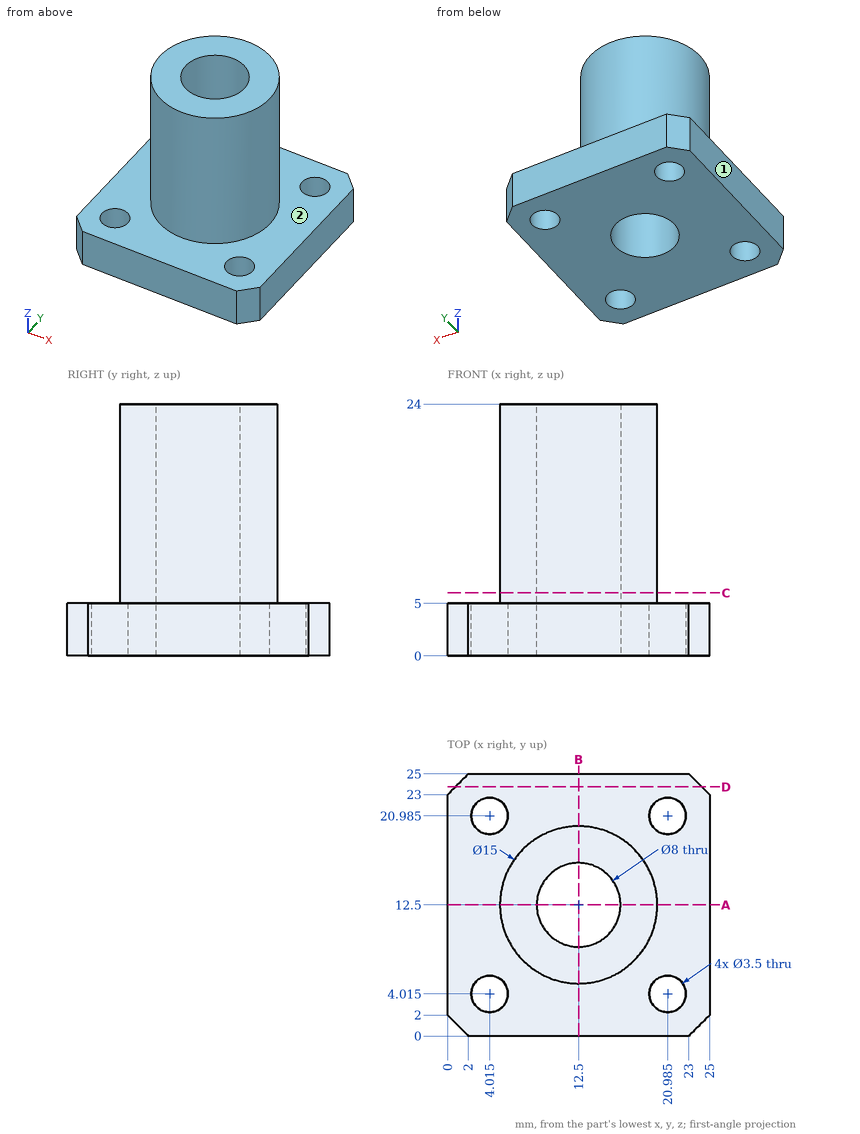
Could you check a few things on this drawing? It's one solid part, dimensions in mm from its lowest x, y, z. A direction names the side the tool comes from. Coordinates: 2 decimals unless noted, no trailing zeros. Order: outer loops, then holes, each group sorted by start corner. A loop starts at its lowest first (then second) coordinate and runs counter-clockwise, first axis right, second up. Notation, with made-up numbers: (-11.5, -10) - (-2.5, -10) arc R15 ccw to (-2.5, 16) - close; hole circle Ø9 at (-5, -8.5). An arc over 180 degrees is marked (long way). Answer as a JSON object with one key per item and string values. Group by question number.
Q1. Imagine slicing it at C-C (z = 6). Please give me the cut outline in (x, y), and give its area (3 significant figures).
Q2. On a 3-axis mill with a long thin cutter (end or side, diameter ignored), from which of +Z, -Z, +X, -X, +Y, -Y can I reach the whole of each face in a straight line? I mean the marked faces 1 and 2. Say none if no direction works.
Q3. I need wall thicknesses on line 1 (Y direction, x = 12.5, z = 13); line 2 (Z direction, x = 4.5, y = 15); line 3 (Y direction, x = 9.75, z = 6) (1 decimal). Which ranges of each line are inside material? Lowest first, please. Write a range as from..to.
Q4. Imagine slicing it at D-D (y = 23.75). Please give me the cut outline in (x, z).
Q5. Will these pins go through, and if not, where does the flat tip stop? P1, Ø5, axis at y = 6.5, z = 20.5, coming from the +X side; P2, Ø8, axis at x = 7.5, y = 5.5, coming from the -Z side; P3, Ø2, axis at x = 15.5, z = 12.5, coming from the -Y side; P4, Ø2, axis at x = 11.5, z = 6.5, coming from the +Y side.
Q6. Imagine slicing it at A-A (y = 12.5). Please give me the cut outline in (x, z), and give its area (3 significant figures).
Determined:
{
 "1": {"outline": "circle Ø15 at (12.5, 12.5); hole circle Ø8 at (12.5, 12.5)", "area": "126 mm2"},
 "2": {"face 1": "+Z, -Z, -X, +Y, -Y", "face 2": "+Z"},
 "3": {"line 1": "y = 5..8.5, 16.5..20", "line 2": "z = 0..5", "line 3": "y = 5.5..9.6, 15.4..19.5"},
 "4": {"outline": "(0.75, 0) - (24.25, 0) - (24.25, 5) - (0.75, 5) - close"},
 "5": {"P1": "stops at x = 19.13", "P2": "stops at z = 0", "P3": "stops at y = 5.27", "P4": "stops at y = 20"},
 "6": {"outline": "(0, 0) - (8.5, 0) - (8.5, 24) - (5, 24) - (5, 5) - (0, 5) - close; (16.5, 0) - (25, 0) - (25, 5) - (20, 5) - (20, 24) - (16.5, 24) - close", "area": "218 mm2"}
}
